from build123d import *

# Parameters (mm, degrees)
F0_W     = 44.45
F0_H     = 124.46
F0_W_2   = 18.415
F0_H_2   = 32.385
F1_DEPTH = 5.08
F0_W_3   = 5.08
F2_DEPTH = 25.4
F3_DEPTH = 19.05


with BuildPart() as f1:
    # F0 (on Front) → F1 (new body)
    with BuildSketch(Plane.XZ):
        with Locations((5.507742, 0.507997)):
            Rectangle(F0_W, F0_H)
        with Locations((5.507742, 0.507997)):
            Rectangle(F0_W_2, F0_H_2, mode=Mode.SUBTRACT)
    extrude(amount=F1_DEPTH)

    # F0 (on Front) → F2 (join)
    with BuildSketch(Plane.XZ):
        with Locations((30.272742, 0.507997)):
            Rectangle(F0_W_3, F0_H)
        with Locations((-19.257258, 0.507997)):
            Rectangle(F0_W_3, F0_H)
    extrude(amount=F2_DEPTH)

    # F0 (on Front) → F3 (join)
    with BuildSketch(Plane.XZ):
        with Locations((5.507742, 0.507997)):
            Rectangle(F0_W_2, F0_H_2)
    extrude(amount=F3_DEPTH)


solid = f1.part
Here's how the part is built. I have some questions about the finished solid (model axes, mm). A direction names the side the tool comes from. Give positions to 0.01 mm unless a question says otherwise; leave off trailing zeros. Write each loop counter-clockwise with the first axis right and the second up, starting at its lowest first coordinate (ties: lowest second). Pieces come first, ordered by that corner, then holes. Notation, with made-up numbers: (57, -23) -> (111, -23) arc R27 ccw to (111, 6) -> close; hole circle Ø1 at (14, 8.5). An arc over 180 degrees is marked (long way). Use one line per item in the form item = value. Start each with the question number.
1. Imagine slicing it at D-D on x = 12.5. List the corners of the cut face in (y, z) for me, plus the area to 3 significant figures.
2. Imagine slicing it at C-C on y = -23.25. List the corners of the cut face in (x, z) for me.
3. Thinking about a two-plate mould opening in X: for faces 1 (the face through (-21.797, -13, 0)), 2 (the face through (-19, -25.4, 1)), 3 (the face through (5, -12, -15.685)), which applies, +X half, -X half, draft (parallel to the pull), parting line (faces both ways), or undercut?
4. If I drill on L1, parallel to X at y = -13.75, z = 13.5; L2, parallel to X at y = -19.5, z = -21; L3, parallel to Y at x = -9.5, z = 28.5, over which ranges is the centre line in solid material (lowest first)?
5. On a 3-axis mill with a long thin cutter (end or side, diameter ignored), from which of +Z, -Z, +X, -X, +Y, -Y can I reach the whole of each face in a straight line? I mean faces 4 (the face through (-16.717, -15, 0)), 5 (the face through (5, 0, 1)), 6 (the face through (5, -12, 16.7)). Say none if no direction works.
6. Will these pins go through, and if not, where does the flat tip stop? pin 1 Ø1 at (x, y) = (-3.5, -7) entering from -Z; pin 2 Ø13.5 at (x, z) = (11.5, -9) entering from -Y; pin 3 Ø4 at (x, y) = (6, -10) entering from +Z.
7. Imagine slicing it at B-B on z = -13. List the corners of the cut face in (x, y) for me, plus the area to 3 significant figures.
8. Imagine slicing it at A-A on y = -10.5. List the corners of the cut face in (x, z) for me, plus the area to 3 significant figures.
Entries:
q1.outline = (-19.05, -15.68) -> (-5.08, -15.68) -> (-5.08, -61.72) -> (0, -61.72) -> (0, 62.74) -> (-5.08, 62.74) -> (-5.08, 16.7) -> (-19.05, 16.7) -> close
q1.area = 1,080 mm²
q2.outline = (-21.8, -61.72) -> (-16.72, -61.72) -> (-16.72, 62.74) -> (-21.8, 62.74) -> close; (27.73, -61.72) -> (32.81, -61.72) -> (32.81, 62.74) -> (27.73, 62.74) -> close
q3.face_1 = -X half
q3.face_2 = draft
q3.face_3 = undercut
q4.L1 = -21.8 to -16.72, -3.7 to 14.72, 27.73 to 32.81
q4.L2 = -21.8 to -16.72, 27.73 to 32.81
q4.L3 = -5.08 to 0
q5.face_4 = +Z, -Z, -Y
q5.face_5 = +Z, -Z, +X, -X, +Y
q5.face_6 = +Z, -Y
q6.pin_1 = -15.68
q6.pin_2 = -19.05
q6.pin_3 = 16.7
q7.outline = (-21.8, -25.4) -> (-16.72, -25.4) -> (-16.72, -5.08) -> (-3.7, -5.08) -> (-3.7, -19.05) -> (14.72, -19.05) -> (14.72, -5.08) -> (27.73, -5.08) -> (27.73, -25.4) -> (32.81, -25.4) -> (32.81, 0) -> (-21.8, 0) -> close
q7.area = 741 mm²
q8.outline = (-21.8, -61.72) -> (-16.72, -61.72) -> (-16.72, 62.74) -> (-21.8, 62.74) -> close; (-3.7, -15.68) -> (14.72, -15.68) -> (14.72, 16.7) -> (-3.7, 16.7) -> close; (27.73, -61.72) -> (32.81, -61.72) -> (32.81, 62.74) -> (27.73, 62.74) -> close
q8.area = 1,860 mm²
